```python
from build123d import *

# Parameters (mm, degrees)
F1_ANGLE_BACK = 60
F1_ANGLE      = 120
F2_T          = -5


with BuildPart() as f1:
    # F0 (on Top) → F1 (revolve)
    with BuildSketch(Plane.XY, mode=Mode.PRIVATE) as f1_sk:
        with BuildLine():
            Line((-12.6999996577, 50.8), (-76.2, 50.8))
            Line((-76.2, 50.8), (-76.2, -12.6999997152))
            ThreePointArc((-76.2, -12.6999997152), (-57.6012803836, 32.2012808271), (-12.6999996577, 50.8))
        make_face()
        with BuildLine():
            ThreePointArc((50.8, -12.7), (32.2012807264, 32.2012804843), (-12.6999996577, 50.8))
            ThreePointArc((-12.6999996577, 50.8), (-57.6012803836, 32.2012808271), (-76.2, -12.6999997152))
            ThreePointArc((-76.2, -12.6999997152), (-12.7000001424, -76.2), (50.8, -12.7))
        make_face()
    revolve(f1_sk.sketch.rotate(Axis((177.8, -25.4, 0), (0, -1, 0)), -F1_ANGLE_BACK), axis=Axis((177.8, -25.4, 0), (0, -1, 0)), revolution_arc=F1_ANGLE)

    # F2
    f2_openings = [f1.faces().sort_by_distance(p)[0] for p in [
        (80.973313, -9.546627, 167.708741),
        (80.973313, -9.546627, -167.708741),
    ]]
    offset(amount=F2_T, openings=f2_openings, kind=Kind.INTERSECTION)

    # F4: F1 across plane


with BuildPart() as f1_1:
    add(f1.part)
    add(f1.part.mirror(Plane(origin=(-7.2496055577, 50.8, 0), x_dir=(-1, 0, 0), z_dir=(0, 1, 0))))


solid = f1_1.part
```
Model file for the job. Use its own axes, mm. A direction names the side the tool comes from. Coordinates: 2 decimals unless noted, no trailing zeros. Loops run counter-clockwise (first coordinate to the right, second up) from the corner with the lowest first, then second, coordinate; pieces in that order, holes last. Notation, with made-up numbers: (-5, -18) -> (38, -18) arc R15 cw to (38, 11) -> close; hole circle Ø10 at (71, 78). An arc over 180 degrees is marked (long way). Answer as a JSON object with one key per item and string values.
Q1. Cut at C-C (y = 131). List the corners of the cut face in (x, z), and give its area (3 significant figures).
Report:
{"outline": "(51.92, -218.03) -> (54.52, -213.53) arc R246.57 cw to (54.52, 213.53) -> (51.92, 218.03) arc R251.76 ccw to start; (110.58, -116.42) -> (113.18, -111.92) arc R129.24 cw to (113.18, 111.92) -> (110.58, 116.42) arc R134.43 ccw to start", "area": "4,150 mm2"}
Q2. Pull direction Y, two halves, no side cores. Call faces 3 (the cylindrical face through (-71.173, 85.459, 3.65)), 4 (the flat face through (-23, 45.8, 5)), 5 (the flat face through (80.05, 50.21, 169.31)): released by +Y, released by -Y, zero draft, split by the parting line, or undercut.
Report:
{"face 3": "undercut", "face 4": "undercut", "face 5": "zero draft"}
Q3. Flat gauge pins, fed straight in: P1, Ø5, axis at y = -38, z = 58.5, coming from the -X side; P2, Ø10, axis at x = 42.5, y = 124, coming from the +Z side; P3, Ø5, axis at y = -1.5, z = 7.5, coming from the +X side. Where does each tip first touch, or does it go through?
Report:
{"P1": "stops at x = -65.18", "P2": "stops at z = 217.28", "P3": "stops at x = 50.46"}
Q4. Probe probe 1 along Y at (x, z) = (29, -124); probe 2 along Y at (x, z) = (-10.5, -94); probe 3 along Y at (x, z) = (27.5, 102). List the from-to ranges inside material, lowest first.
Report:
{"probe 1": "y = -76.12 to -71.11, 45.8 to 55.8, 172.71 to 177.72", "probe 2": "y = -72.98 to -67.69, 45.8 to 55.8, 169.29 to 174.58", "probe 3": "y = -75.58 to -70.53, 45.13 to 50.18, 51.42 to 56.47, 172.13 to 177.18"}
Q5. Cut at B-B (x = 102.5). State how many separate pieces and enclosed holes the cut face has, and give its area (3 significant figures).
Report:
{"separate pieces": "4", "enclosed holes": "0", "area": "2,510 mm2"}
Q6. 3-axis set-ups, long thin cutter, end or side, ignore diameter. For faces 1 (the flat face through (-23, 55.8, 5)), 2 (the flat face through (80.05, 50.21, -169.31)): which of +Z, -Z, +X, -X, +Y, -Y reach the whole face in a straight line?
Report:
{"face 1": "none", "face 2": "-Z, +X, +Y, -Y"}
Q7. Cut at A-A (y = 87). List the corners of the cut face in (x, z), and give its area (3 significant figures).
Report:
{"outline": "(50.8, -219.97) -> (53.3, -215.64) arc R249 cw to (53.3, 215.64) -> (50.8, 219.97) arc R254 ccw to start; (108.42, -120.17) -> (111.22, -115.33) arc R133.17 cw to (111.22, 115.33) -> (108.42, 120.17) arc R138.76 ccw to start", "area": "4,230 mm2"}
